Could you check a few things on this model? Use its own coordinates, in mm. A direction names the side the tool comes from. Coordinates: 2 decimals unless noted, no trailing zeros. Loops run counter-clockwise (first coordinate to the right, second up) from the corner with the lowest first, then second, coordinate; pieces in that order, holes last. Notation, with made-up numbers: (-18, -28) - (29, -28) arc R16 cw to (29, -2) - close; hole circle Ø9 at (50, -2.5). An arc over 180 degrees is marked (long way). Use CSV: the item, a comma, the result in double quotes.
from build123d import *

# Parameters (mm, degrees)
SKETCH1_W           = 30
SKETCH1_H           = 30
BOSS_EXTRUDE3_DEPTH = 8
SKETCH3_R           = 4.25
CUT_EXTRUDE2_DEPTH  = 5
FILLET2_R           = 15


with BuildPart() as part:
    # Sketch1 → Boss-Extrude3 (new body)
    with BuildSketch(Plane(origin=(0, 0, 0), x_dir=(1, 0, 0), z_dir=(0, 1, 0))):
        with Locations((-4.26121372, -7.941952507)):
            Rectangle(SKETCH1_W, SKETCH1_H)
    extrude(amount=BOSS_EXTRUDE3_DEPTH)

    # Sketch3 → Cut-Extrude2 (cut)
    with BuildSketch(Plane(origin=(0, 8, 0), x_dir=(1, 0, 0), z_dir=(0, 1, 0))):
        with Locations(Location((-4.26121372, -7.941952507, 0), (0, 0, 270))):
            Circle(SKETCH3_R)
    extrude(amount=-CUT_EXTRUDE2_DEPTH, mode=Mode.SUBTRACT)

    # Fillet2
    fillet2_edges = [part.edges().sort_by_distance(p)[0] for p in [
        (10.73878628, 4, 22.941952507),
        (-19.26121372, 4, 22.941952507),
        (-19.26121372, 4, -7.058047493),
        (10.73878628, 4, -7.058047493),
    ]]
    fillet(fillet2_edges, radius=FILLET2_R - 0.0001)  # a hair under: the kernel refuses the full size


solid = part.part
(1) Thinking about a two-plate mould opening in X: for faces 3 (the face through (-0.047, 5.535, 7.389)), 4 (the face through (-4, 0, 8)), 5 (the face through (6, 4, -3)), which applies, +X half, -X half, draft (parallel to the pull), parting line (faces both ways), or undercut?
Computed:
face 3,"undercut"
face 4,"draft"
face 5,"+X half"
(2) Suppose I cut it at C-C (z = 10.5). Write out the boundary of the cut face in (x, y).
Computed:
outline,"(-19.04, 0) - (10.52, 0) - (10.52, 8) - (-0.87, 8) - (-0.87, 3) - (-7.66, 3) - (-7.66, 8) - (-19.04, 8) - close"
(3) Please list where these lines run through material, in increasing order: line 1 (Z direction, x = -5, y = 5.5); line 2 (X direction, y = 4, z = 11); line 3 (X direction, y = 6.25, z = -4).
Computed:
line 1,"z = -7.04 to 3.76, 12.13 to 22.92"
line 2,"x = -18.95 to -7.21, -1.31 to 10.42"
line 3,"x = -13.34 to 4.82"
(4) Which directions (+Z, -Z, +X, -X, +Y, -Y) give clear straight access to the entire face, cutting with the end or side of a thin tool? Please do faces 1 (the face through (-14.984, 4.056, 18.431)), 2 (the face through (-4, 3, 8)).
Computed:
face 1,"+Z, -X, +Y, -Y"
face 2,"+Y"
(5) Will these pins go through, and if not, where does the flat tip stop? pin 1 (4 mm diameter, centred on x = -6, z = 7.5, fed in from +Y); pin 2 (4 mm diameter, centred on x = 5, y = 1, fed in from +Z).
Computed:
pin 1,"stops at y = 3"
pin 2,"stops at z = 21.07"
(6) Suppose I cut it at D-D (z = -3). Write out the boundary of the cut face in (x, y), plus the area to 3 significant figures.
Computed:
outline,"(-14.52, 0) - (6, 0) - (6, 8) - (-14.52, 8) - close"
area,"164 mm²"
(7) Suppose I cut it at B-B (x = -2). Write out the boundary of the cut face in (y, z), plus the area to 3 significant figures.
Computed:
outline,"(0, -6.89) - (8, -6.89) - (8, 4.34) - (3, 4.34) - (3, 11.54) - (8, 11.54) - (8, 22.77) - (0, 22.77) - close"
area,"201 mm²"
